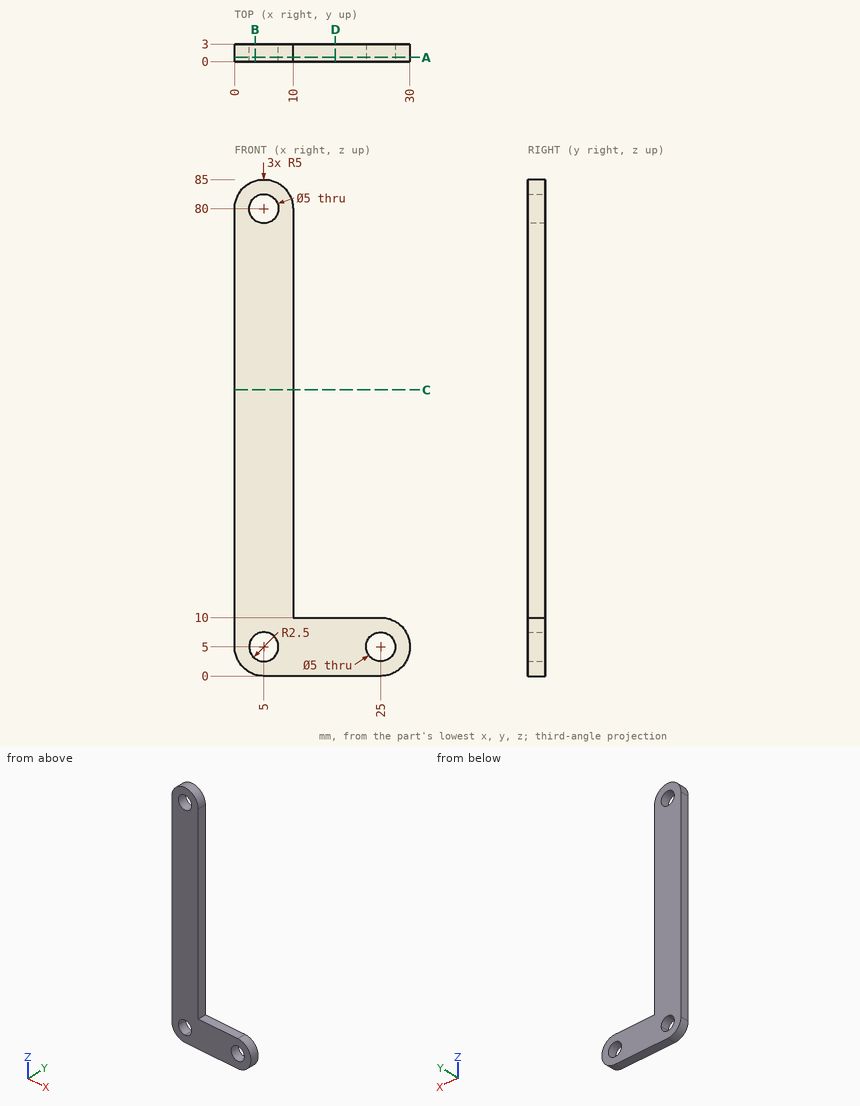
Can you work these out from the drawing? Everything is in mm from the part's minimum corner. Coordinates: 2 decimals unless noted, no trailing zeros. Loops run counter-clockwise (first coordinate to the right, second up) from the corner with the lowest first, then second, coordinate; pieces in that order, holes last. Notation, with made-up numbers: M -10,22 L 1,22 A9 cw 1,32 Z; hole C 9,-32.75 d11. An arc over 180 degrees is marked long. One line per item, written item: value.
1. Will these pins go through, and if not, where does the flat tip stop? pin 1 Ø1 at (x, y) = (13, 2.5) entering from +Z; pin 2 Ø3 at (x, z) = (8.5, 25) entering from -Y; pin 3 Ø0.9 at (y, z) = (1.5, 36) entering from +X.
Geometry says:
pin 1: stops at z = 10
pin 2: stops at y = 0
pin 3: stops at x = 10
2. Imagine slicing it at D-D (x = 17.25). List the corners of the cut face in (y, z) for me.
Geometry says:
outline: M 0,0 L 3,0 L 3,10 L 0,10 Z
3. Imagine slicing it at C-C (z = 49). List the corners of the cut face in (x, y) for me, and give its area (3 significant figures).
Geometry says:
outline: M 0,0 L 10,0 L 10,3 L 0,3 Z
area: 30.0 mm2
4. Imagine slicing it at A-A (y = 0.7). List the corners of the cut face in (x, z) for me, and give its area (3 significant figures).
Geometry says:
outline: M 0,5 A5 ccw 5,0 L 25,0 A5 ccw 25,10 L 10,10 L 10,80 A5 ccw 0,80 Z; hole C 5,5 d5; hole C 5,80 d5; hole C 25,5 d5
area: 964 mm2
5. Imagine slicing it at B-B (x = 3.5). List the corners of the cut face in (y, z) for me.
Geometry says:
outline: M 0,0.23 L 3,0.23 L 3,3 L 0,3 Z; M 0,7 L 3,7 L 3,78 L 0,78 Z; M 0,82 L 3,82 L 3,84.77 L 0,84.77 Z
6. Please list where these lines run through material, in increasing order: probe 1 along X at (y, z) = (1.1, 5); probe 2 along X at (y, z) = (1.95, 80); probe 3 along Z at (x, y) = (2.75, 0.9).
Geometry says:
probe 1: x = 0 to 2.5, 7.5 to 22.5, 27.5 to 30
probe 2: x = 0 to 2.5, 7.5 to 10
probe 3: z = 0.53 to 3.91, 6.09 to 78.91, 81.09 to 84.47
